```python
from build123d import *

# Parameters (mm, degrees)
BOSS_EXTRUDE1_DEPTH = 104
SKETCH2_W           = 34
SKETCH2_H           = 10
CUT_EXTRUDE1_DEPTH  = 2
CUT_EXTRUDE2_REACH  = 141.82
SKETCH3_W           = 100
SKETCH3_H           = 52


with BuildPart() as part:
    # Sketch1 → Boss-Extrude1 (new body)
    with BuildSketch(Plane(origin=(0, 0, 0), x_dir=(0, 0, -1), z_dir=(1, 0, 0))):
        Polygon((0, 0), (93, 0), (93, 2), (2, 2), (2, 9.2), (10, 9.2), (10, 11.2), (0, 11.2), align=None)
    extrude(amount=BOSS_EXTRUDE1_DEPTH)

    # Sketch2 → Cut-Extrude1 (cut)
    with BuildSketch(Plane(origin=(0, 11.2, 0), x_dir=(1, 0, 0), z_dir=(0, 1, 0))):
        with Locations((67, 5)):
            Rectangle(SKETCH2_W, SKETCH2_H)
    extrude(amount=-CUT_EXTRUDE1_DEPTH, mode=Mode.SUBTRACT)

    # Sketch3 → Cut-Extrude2 (cut, up to next)
    with BuildSketch(Plane(origin=(0, 2, 0), x_dir=(1, 0, 0), z_dir=(0, 1, 0)), mode=Mode.PRIVATE) as cut_extrude2_sk1:
        with Locations((52, 54)):
            Rectangle(SKETCH3_W, SKETCH3_H)
    cut_extrude2_tool1 = extrude(cut_extrude2_sk1.sketch, amount=-CUT_EXTRUDE2_REACH, mode=Mode.PRIVATE) & part.part
    add(cut_extrude2_tool1.solids().sort_by_distance((52, 2, -54))[0], mode=Mode.SUBTRACT)


solid = part.part
```
Verification items for the finished model (mm, model axes). A direction names the side the tool comes from. Coordinates: 2 decimals unless noted, no trailing zeros. Loops run counter-clockwise (first coordinate to the right, second up) from the corner with the lowest first, then second, coordinate; pieces in that order, holes last. Notation, with made-up numbers: (41, 38) - (55, 38) arc R22 ccw to (55, 52) - close; hole circle Ø7 at (82.5, -7.5). An arc over 180 degrees is marked (long way). Return JSON: item names as keys, results as strings.
1. Tool access check on faces 5 (the flat face through (0, 1, -36)), 6 (the flat face through (51, 6, -2)). Record the directions out of +Z, -Z, +X, -X, +Y, -Y that give a thin tool (end or side, any length) a straight path to the whole face; none if there is none.
Established:
{"face 5": "+Z, -Z, -X, +Y, -Y", "face 6": "-Z, +X, -X"}
2. Section check D-D, the plane y = 6.75. Record the boundary of the cut face in (x, z).
Established:
{"outline": "(0, -2) - (104, -2) - (104, 0) - (0, 0) - close"}
3. Mould release check, pull along Y, two halves, no side actions. Record for faces 1 (the flat face through (94, 9.2, -6)), 2 (the flat face through (51, 6, 0)), 3 (the flat face through (94, 11.2, -5)), 4 (the flat face through (25, 9.2, -6)): +Y half, -Y half, draft (parallel to the pull), parting line (faces both ways), or undercut.
Established:
{"face 1": "undercut", "face 2": "draft", "face 3": "+Y half", "face 4": "undercut"}
4. Go/stop test with flat-tipped pins: pin 1 (6 mm diameter, centred on y = 2, z = -70.5, fed in from -X); pin 2 (0.6 mm diameter, centred on x = 98.5, y = 10.5, fed in from -Z); pin 3 (3 mm diameter, centred on x = 83, z = -12.5, fed in from +Y); pin 4 (2 mm diameter, centred on x = 74.5, z = -0.5, fed in from +Y). Record where each tip stops, or that it passes through.
Established:
{"pin 1": "stops at x = 0", "pin 2": "stops at z = -10", "pin 3": "stops at y = 2", "pin 4": "stops at y = 9.2"}
5. Section check C-C, the plane x = 75.5. Record the boundary of the cut face in (y, z).
Established:
{"outline": "(0, -93) - (2, -93) - (2, -80) - (0, -80) - close; (0, -28) - (2, -28) - (2, -2) - (9.2, -2) - (9.2, 0) - (0, 0) - close"}
6. Thickness scan on L1, parallel to Y at x = 46.5, z = -9; L2, parallel to X at y = 1, z = -78.5; L3, parallel to Z at x = 38, y = 8. Record the ranges inside material, lowest first.
Established:
{"L1": "y = 0 to 2, 9.2 to 11.2", "L2": "x = 0 to 2, 102 to 104", "L3": "z = -2 to 0"}
7. Section check A-A, the plane x = 34. Record the boundary of the cut face in (y, z).
Established:
{"outline": "(0, -93) - (2, -93) - (2, -80) - (0, -80) - close; (0, -28) - (2, -28) - (2, -2) - (9.2, -2) - (9.2, -10) - (11.2, -10) - (11.2, 0) - (0, 0) - close"}
8. Section check B-B, the plane z = -78. Record the boundary of the cut face in (x, y), then the cut area to 3 significant figures.
Established:
{"outline": "(0, 0) - (2, 0) - (2, 2) - (0, 2) - close; (102, 0) - (104, 0) - (104, 2) - (102, 2) - close", "area": "8.00 mm2"}
